Read the model definition and answer for the solid it produces. Units are mm, in the model's axes. A direction names the side the tool comes from. Coordinates: 2 decimals unless noted, no trailing zeros. Loops run counter-clockwise (first coordinate to the right, second up) from the corner with the lowest first, then second, coordinate; pieces in that order, holes last. Notation, with made-up numbers: (68, 27) -> (74, 27) arc R35 ccw to (74, 60) -> close; hole circle Ø6 at (86.25, -10.5). An arc over 180 degrees is marked (long way). Answer as a JSON object with one key per item and string values. Group by question number.
Q1. For faces 1 (the flat face through (-8, -8.9, 99)), 2 (the flat face through (-22.5, 3, 49)), 3 (the flat face through (-8, -6.1, 99)), determine the directions among +Z, -Z, +X, -X, +Y, -Y from which every point of the face is accessible in a straight line to the end or side of a thin tool.
Q2. Straight lines are drawn through the part: line 1 along X through (y, z) = (1.25, 78.5); line 2 along Z through (x, y) = (-4, 8.25); line 3 along X through (y, z) = (-5.5, 36.5). For each, find the intervals that lie inside material, in ascending order. Write a range as [from, to].
Q3. The part is cut by section B-B on z = 22. Write down the section's boundary in (x, y).
Q4. Each of these flat-tipped pins is pushed along its axis until it touches: P1, Ø2, axis at x = -1, z = 48.5, coming from the +Y side; P2, Ø6.5, axis at y = -0.5, z = 40.5, coming from the +X side. Where does it stop, or does it pass through?
Q5. The part is cut by section A-A on y = 8.25. State how many separate pieces and enclosed holes the cut face has, and give its area (4 significant figures).
Q6. Determine the mould class of faces 4 (the flat face through (24, 9, 49)), 5 (the flat face through (0, -1, 0)), 6 (the flat face through (16, 7.1, 99)) for opening direction X: released by +X, released by -X, zero draft, split by the parting line, or undercut.
from build123d import *

# Parameters (mm, degrees)
RESSALTO_EXTRUS_O1_DEPTH = 100
RESSALTO_EXTRUS_O3_REACH = 107.835
ESBO_O3_W                = 45
ESBO_O3_H                = 1.5
CORTE_EXTRUS_O1_DEPTH    = 103.343783397
ESBO_O5_W                = 12
ESBO_O5_H                = 1.5
CORTE_EXTRUS_O2_DEPTH    = 106.834776893
ESBO_O6_W                = 45
ESBO_O6_H                = 2
RESSALTO_EXTRUS_O4_DEPTH = 25
ESBO_O7_W                = 2.8
ESBO_O7_H                = 2.8
CORTE_EXTRUS_O3_DEPTH    = 10
CORTE_EXTRUS_O4_DEPTH    = 104.788245963
RESSALTO_EXTRUS_O5_DEPTH = 100
ESBO_O10_W               = 0.5
ESBO_O10_H               = 8
CORTE_EXTRUS_O5_DEPTH    = 104.788245963
CHANFRO1_SIZE            = 3
CHANFRO2_SIZE            = 3


with BuildPart() as part:
    # Esboço1 → Ressalto-extrusão1 (new body)
    with BuildSketch(Plane.XY):
        Polygon((-22.5, 12.5), (-22.5, -7.5), (-17.5, -12.5), (17.5, -12.5), (22.5, -7.5), (22.5, 12.5), (24, 12.5), (24, -9), (19, -14), (-19, -14), (-24, -9), (-24, 12.5), align=None)
    extrude(amount=RESSALTO_EXTRUS_O1_DEPTH)

    # Ressalto-extrusão3: up to this face of the body (flat: up to its plane)
    ressalto_extrus_o3_end = Plane(part.part.faces().sort_by_distance((-23.25, 12.5, 50))[0])
    # Esboço3 → Ressalto-extrusão3 (add, up to the picked face)
    with BuildSketch(Plane(origin=(0, -12.5, 0), x_dir=(1, 0, 0), z_dir=(0, 1, 0)), mode=Mode.PRIVATE) as ressalto_extrus_o3_sk1:
        with Locations((0, -0.75)):
            Rectangle(ESBO_O3_W, ESBO_O3_H)
    ressalto_extrus_o3_tool1 = split(extrude(ressalto_extrus_o3_sk1.sketch, amount=RESSALTO_EXTRUS_O3_REACH, mode=Mode.PRIVATE), bisect_by=ressalto_extrus_o3_end, keep=Keep.BOTH, mode=Mode.PRIVATE)
    add(ressalto_extrus_o3_tool1.solids().sort_by(Axis((0, -12.5, 0.75), (0, 1, 0)))[0])

    # Esboço4 → Corte-extrusão1 (cut, through all)
    with BuildSketch(Plane.XY.offset(1.5)):
        Polygon((-10, -12.5), (10, -12.5), (10, -7.5), (5, -2.5), (-5, -2.5), (-10, -7.5), align=None)
    extrude(amount=-CORTE_EXTRUS_O1_DEPTH, mode=Mode.SUBTRACT)

    # Esboço5 → Corte-extrusão2 (cut, through all)
    with BuildSketch(Plane(origin=(0, -12.5, 0), x_dir=(1, 0, 0), z_dir=(0, 1, 0))):
        with Locations((0, -2.25)):
            Rectangle(ESBO_O5_W, ESBO_O5_H)
    extrude(amount=-CORTE_EXTRUS_O2_DEPTH, mode=Mode.SUBTRACT)

    # Esboço6 → Ressalto-extrusão4 (add)
    with BuildSketch(Plane(origin=(0, -12.5, 0), x_dir=(1, 0, 0), z_dir=(0, 1, 0))):
        with Locations((0, -99)):
            Rectangle(ESBO_O6_W, ESBO_O6_H)
    extrude(amount=RESSALTO_EXTRUS_O4_DEPTH)

    # Esboço7 → Corte-extrusão3 (cut)
    with BuildSketch(Plane.XY.offset(100)):
        with Locations((-8, 8.5)):
            Rectangle(ESBO_O7_W, ESBO_O7_H)
        with Locations((-16, 8.5)):
            Rectangle(ESBO_O7_W, ESBO_O7_H)
        with Locations((0, 8.5)):
            Rectangle(ESBO_O7_W, ESBO_O7_H)
        with Locations((8, 8.5)):
            Rectangle(ESBO_O7_W, ESBO_O7_H)
        with Locations((16, 8.5)):
            Rectangle(ESBO_O7_W, ESBO_O7_H)
        with Locations((-8, 0.5)):
            Rectangle(ESBO_O7_W, ESBO_O7_H)
        with Locations((0, 0.5)):
            Rectangle(ESBO_O7_W, ESBO_O7_H)
        with Locations((8, 0.5)):
            Rectangle(ESBO_O7_W, ESBO_O7_H)
        with Locations((16, 0.5)):
            Rectangle(ESBO_O7_W, ESBO_O7_H)
        with Locations((-8, -7.5)):
            Rectangle(ESBO_O7_W, ESBO_O7_H)
        with Locations((0, -7.5)):
            Rectangle(ESBO_O7_W, ESBO_O7_H)
        with Locations((8, -7.5)):
            Rectangle(ESBO_O7_W, ESBO_O7_H)
        with Locations((16, -7.5)):
            Rectangle(ESBO_O7_W, ESBO_O7_H)
        with Locations((-16, 0.5)):
            Rectangle(ESBO_O7_W, ESBO_O7_H)
        with Locations((-16, -7.5)):
            Rectangle(ESBO_O7_W, ESBO_O7_H)
    extrude(amount=-CORTE_EXTRUS_O3_DEPTH, mode=Mode.SUBTRACT)

    # Esboço8 → Corte-extrusão4 (cut, through all)
    with BuildSketch(Plane(origin=(0, 0, 0), x_dir=(-1, 0, 0), z_dir=(0, 0, -1))):
        Polygon((-22.5, -10.5), (-22.5, -12.5), (-20.5, -12.5), align=None)
        Polygon((20.5, -12.5), (22.5, -12.5), (22.5, -10.5), align=None)
    extrude(amount=-CORTE_EXTRUS_O4_DEPTH, mode=Mode.SUBTRACT)

    # Esboço9 → Ressalto-extrusão5 (add, through all)
    with BuildSketch(Plane(origin=(0, 0, 0), x_dir=(-1, 0, 0), z_dir=(0, 0, -1))):
        Polygon((-19, -14), (-21.5, -14), (-21.5, -11.5), align=None)
        Polygon((19, -14), (21.5, -14), (21.5, -11.5), align=None)
    extrude(amount=-RESSALTO_EXTRUS_O5_DEPTH)

    # Esboço10 → Corte-extrusão5 (cut, through all)
    with BuildSketch(Plane(origin=(0, 0, 0), x_dir=(-1, 0, 0), z_dir=(0, 0, -1))):
        with Locations((-23.75, 0.5)):
            Rectangle(ESBO_O10_W, ESBO_O10_H)
        with Locations((23.75, 0.5)):
            Rectangle(ESBO_O10_W, ESBO_O10_H)
    extrude(amount=-CORTE_EXTRUS_O5_DEPTH, mode=Mode.SUBTRACT)

    # Chanfro1
    # the kernel refuses this chamfer: 3 mm, written as the material it adds along each edge
    with BuildSketch(Plane(origin=(22.5, -15.215048964, 98), x_dir=(0.027495876610586768, 0, -0.9996219169112968), z_dir=(0, 1, 0))) as chanfro1_piece_1_section:
        Polygon((CHANFRO1_SIZE * 0.999621916911, CHANFRO1_SIZE * 0.0274958766106), (-CHANFRO1_SIZE * 0.0274958766106, CHANFRO1_SIZE * 0.999621916911), (0, 0), align=None)
    chanfro1_piece_1 = extrude(amount=27.715048964, mode=Mode.PRIVATE)
    chanfro1_piece_1 = split(chanfro1_piece_1, bisect_by=Plane(origin=(27.146986971, -2.853013029, 96.73534202), z_dir=(-0.7071067811865475, 0.7071067811865476, 0)), keep=Keep.TOP, mode=Mode.PRIVATE)
    add(chanfro1_piece_1)
    with BuildSketch(Plane(origin=(12.04463656, -17.95536344, 98), x_dir=(-0.7068394360706735, 0.7068394360706735, 0.027495876610586778), z_dir=(0.7071067811865476, 0.7071067811865475, 0))) as chanfro1_piece_2_section:
        Polygon((CHANFRO1_SIZE * 0.999621916911, -CHANFRO1_SIZE * 0.0274958766106), (-CHANFRO1_SIZE * 0.0274958766106, -CHANFRO1_SIZE * 0.999621916911), (0, 0), align=None)
    chanfro1_piece_2 = extrude(amount=22.50116574, mode=Mode.PRIVATE)
    chanfro1_piece_2 = split(chanfro1_piece_2, bisect_by=Plane(origin=(16.362312496, -12.5, 97.266244129), z_dir=(0, 1, 0)), keep=Keep.TOP, mode=Mode.PRIVATE)
    chanfro1_piece_2 = split(chanfro1_piece_2, bisect_by=Plane(origin=(16.362312496, -8.9, 97.266244129), z_dir=(0, -1, 0)), keep=Keep.TOP, mode=Mode.PRIVATE)
    add(chanfro1_piece_2)
    with BuildSketch(Plane(origin=(12.04463656, -17.95536344, 98), x_dir=(-0.7068394360706735, 0.7068394360706735, 0.027495876610586778), z_dir=(0.7071067811865476, 0.7071067811865475, 0))) as chanfro1_piece_3_section:
        Polygon((CHANFRO1_SIZE * 0.999621916911, -CHANFRO1_SIZE * 0.0274958766106), (-CHANFRO1_SIZE * 0.0274958766106, -CHANFRO1_SIZE * 0.999621916911), (0, 0), align=None)
    chanfro1_piece_3 = extrude(amount=22.50116574, mode=Mode.PRIVATE)
    chanfro1_piece_3 = split(chanfro1_piece_3, bisect_by=Plane(origin=(22.5, -7.314063038, 97.124733651), z_dir=(-1, 0, 0)), keep=Keep.TOP, mode=Mode.PRIVATE)
    chanfro1_piece_3 = split(chanfro1_piece_3, bisect_by=Plane(origin=(17.4, -7.314063038, 97.124733651), z_dir=(1, 0, 0)), keep=Keep.TOP, mode=Mode.PRIVATE)
    add(chanfro1_piece_3)
    with BuildSketch(Plane(origin=(25.215048964, -12.5, 98), x_dir=(0, -0.02749587661058619, -0.9996219169112968), z_dir=(-1, 0, 0))) as chanfro1_piece_4_section:
        Polygon((CHANFRO1_SIZE * 0.999621916911, -CHANFRO1_SIZE * 0.0274958766106), (-CHANFRO1_SIZE * 0.0274958766106, -CHANFRO1_SIZE * 0.999621916911), (0, 0), align=None)
    chanfro1_piece_4 = extrude(amount=50.430097928, mode=Mode.PRIVATE)
    chanfro1_piece_4 = split(chanfro1_piece_4, bisect_by=Plane(origin=(-9.263513514, -20.736486486, 97.013513514), z_dir=(0.7071067811865475, 0.7071067811865476, 0)), keep=Keep.TOP, mode=Mode.PRIVATE)
    chanfro1_piece_4 = split(chanfro1_piece_4, bisect_by=Plane(origin=(9.263513514, -20.736486486, 97.013513514), z_dir=(-0.7071067811865475, 0.7071067811865476, 0)), keep=Keep.TOP, mode=Mode.PRIVATE)
    add(chanfro1_piece_4)
    with BuildSketch(Plane(origin=(-27.95536344, -2.04463656, 98), x_dir=(0.7068394360706733, 0.7068394360706736, 0.027495876610586757), z_dir=(0.7071067811865476, -0.7071067811865475, 0))) as chanfro1_piece_5_section:
        Polygon((CHANFRO1_SIZE * 0.999621916911, -CHANFRO1_SIZE * 0.0274958766106), (-CHANFRO1_SIZE * 0.0274958766106, -CHANFRO1_SIZE * 0.999621916911), (0, 0), align=None)
    chanfro1_piece_5 = extrude(amount=22.50116574, mode=Mode.PRIVATE)
    chanfro1_piece_5 = split(chanfro1_piece_5, bisect_by=Plane(origin=(-22.5, -3.439339828, 97.957106781), z_dir=(1, 0, 0)), keep=Keep.TOP, mode=Mode.PRIVATE)
    chanfro1_piece_5 = split(chanfro1_piece_5, bisect_by=Plane(origin=(-17.4, -3.439339828, 97.957106781), z_dir=(-1, 0, 0)), keep=Keep.TOP, mode=Mode.PRIVATE)
    add(chanfro1_piece_5)
    with BuildSketch(Plane(origin=(-27.95536344, -2.04463656, 98), x_dir=(0.7068394360706733, 0.7068394360706736, 0.027495876610586757), z_dir=(0.7071067811865476, -0.7071067811865475, 0))) as chanfro1_piece_6_section:
        Polygon((CHANFRO1_SIZE * 0.999621916911, -CHANFRO1_SIZE * 0.0274958766106), (-CHANFRO1_SIZE * 0.0274958766106, -CHANFRO1_SIZE * 0.999621916911), (0, 0), align=None)
    chanfro1_piece_6 = extrude(amount=22.50116574, mode=Mode.PRIVATE)
    chanfro1_piece_6 = split(chanfro1_piece_6, bisect_by=Plane(origin=(-16.362312496, -12.5, 97.266244129), z_dir=(0, 1, 0)), keep=Keep.TOP, mode=Mode.PRIVATE)
    chanfro1_piece_6 = split(chanfro1_piece_6, bisect_by=Plane(origin=(-16.362312496, -8.9, 97.266244129), z_dir=(0, -1, 0)), keep=Keep.TOP, mode=Mode.PRIVATE)
    add(chanfro1_piece_6)
    with BuildSketch(Plane(origin=(-22.5, -15.215048964, 98), x_dir=(-0.027495876610586768, 0, -0.9996219169112968), z_dir=(0, 1, 0))) as chanfro1_piece_7_section:
        Polygon((CHANFRO1_SIZE * 0.999621916911, -CHANFRO1_SIZE * 0.0274958766106), (-CHANFRO1_SIZE * 0.0274958766106, -CHANFRO1_SIZE * 0.999621916911), (0, 0), align=None)
    chanfro1_piece_7 = extrude(amount=27.715048964, mode=Mode.PRIVATE)
    chanfro1_piece_7 = split(chanfro1_piece_7, bisect_by=Plane(origin=(-27.146986971, -2.853013029, 96.73534202), z_dir=(0.7071067811865475, 0.7071067811865476, 0)), keep=Keep.TOP, mode=Mode.PRIVATE)
    add(chanfro1_piece_7)

    # Chanfro2
    chanfro2_edges = [part.edges().sort_by_distance(p)[0] for p in [
        (-13.75, -12.5, 1.5),
        (20, -10, 1.5),
        (-22.5, 2.5, 1.5),
        (-20, -10, 1.5),
        (22.5, 2.5, 1.5),
        (13.75, -12.5, 1.5),
    ]]
    chamfer(chanfro2_edges, length=CHANFRO2_SIZE)


solid = part.part
Final values:
{
 "1": {"face 1": "+Z, -Z", "face 2": "+Y", "face 3": "+Z"},
 "2": {"line 1": "x = [-23.5, -22.5], [22.5, 23.5]", "line 2": "z = [0, 1.5], [98, 100]", "line 3": "x = [-24, -22.5], [22.5, 24]"},
 "3": {"outline": "(-24, -9) -> (-21.5, -11.5) -> (-21.5, -14) -> (21.5, -14) -> (21.5, -11.5) -> (24, -9) -> (24, -3.5) -> (23.5, -3.5) -> (23.5, 4.5) -> (24, 4.5) -> (24, 12.5) -> (22.5, 12.5) -> (22.5, -7.5) -> (17.5, -12.5) -> (-17.5, -12.5) -> (-22.5, -7.5) -> (-22.5, 12.5) -> (-24, 12.5) -> (-24, 4.5) -> (-23.5, 4.5) -> (-23.5, -3.5) -> (-24, -3.5) -> close"},
 "4": {"P1": "stops at y = -12.5", "P2": "stops at x = 24"},
 "5": {"separate pieces": "5", "enclosed holes": "0", "area": "447.5 mm2"},
 "6": {"face 4": "released by +X", "face 5": "zero draft", "face 6": "undercut"}
}
